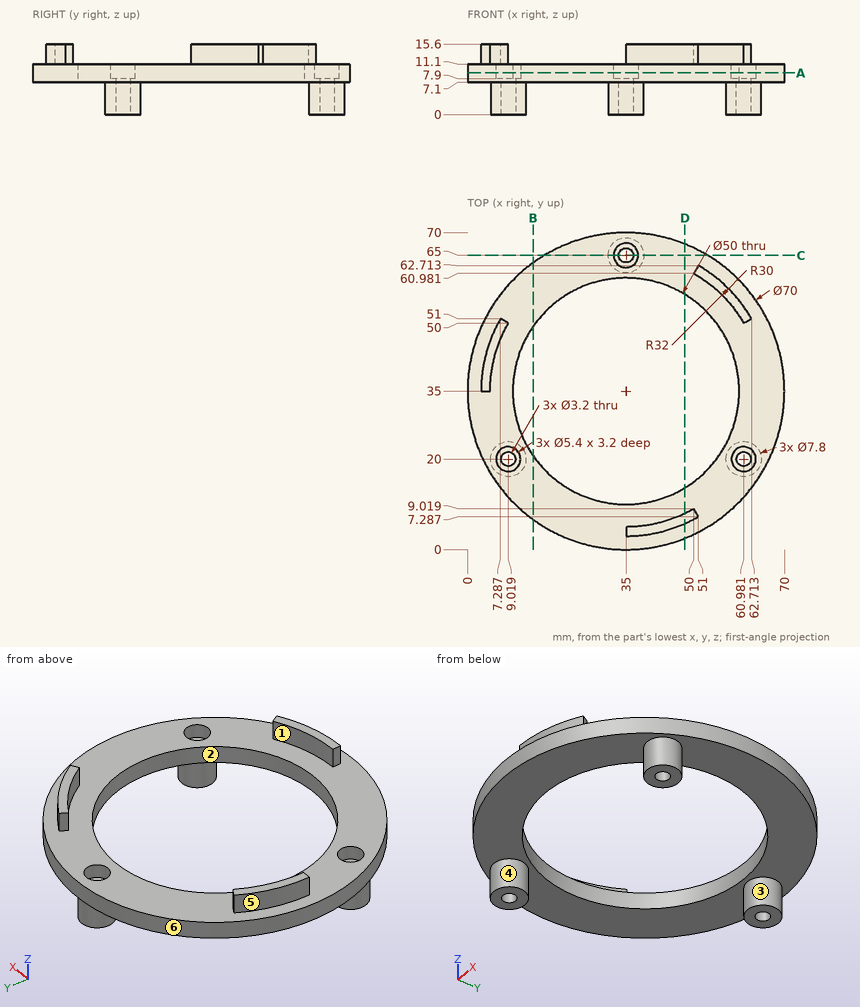
Drawing for the job (mm, zero at the part's lowest x, y, z). A direction names the side the tool comes from. Give positions to 0.01 mm unless a question says otherwise; leave off trailing zeros. Loops run counter-clockwise (first coordinate to the right, second up) from the corner with the lowest first, then second, coordinate; pieces in that order, holes last.
(1) Pin check, flat tips, straight feed: pin 1 (12 mm diameter, centred on x = 36.5, y = 12.5, fed in from +Z); pin 2 (8 mm diameter, centred on y = 45.5, z = 4, fed in from -X); pin 3 (1.6 mm diameter, centred on x = 8.5, y = 19, fed in from +Z). Stop position of each tip, or through.
Return value:
pin 1: stops at z = 11.1
pin 2: stops at x = 0.92
pin 3: stops at z = 7.9
(2) Drill centre lines: line 1 along Y through (x, z) = (35, 9.6); line 2 along Z through (x, y) = (62, 28.5); line 3 along Y through (x, z) = (35, 2.75). Where is each one in solid material? Low to high.
Return value:
line 1: y = 0 to 10, 60 to 62.3, 67.7 to 70
line 2: z = 7.1 to 11.1
line 3: y = 61.1 to 63.4, 66.6 to 68.9
(3) Band-saw the part on C-C (y = 65). Write the cut outline in (x, z).
Return value:
outline: (16.97, 7.1) - (31.1, 7.1) - (31.1, 0) - (33.4, 0) - (33.4, 7.9) - (32.3, 7.9) - (32.3, 11.1) - (16.97, 11.1) - close; (36.6, 0) - (38.9, 0) - (38.9, 7.1) - (53.03, 7.1) - (53.03, 11.1) - (37.7, 11.1) - (37.7, 7.9) - (36.6, 7.9) - close
(4) 3-axis set-ups, long thin cutter, end or side, ignore diameter. For the marked faces 4, 5 and 6: which of +Z, -Z, +X, -X, +Y, -Y reach the whole face in a straight line?
Return value:
face 4: -Z
face 5: +Z, -X, +Y
face 6: +Z, -Z
(5) Band-saw the part on B-B (x = 14.5). Write the cut outline in (y, z).
Return value:
outline: (6.63, 7.1) - (20.69, 7.1) - (20.69, 11.1) - (6.63, 11.1) - close; (49.31, 7.1) - (63.37, 7.1) - (63.37, 11.1) - (49.31, 11.1) - close
(6) Pull direction X, two halves, no side cores. Call the marked faces 1, 2 and 3: pulls with the +X half, pulls with the -X half, needs draft (parallel to the pull), parting line crosses it, or undercut.
Return value:
face 1: pulls with the -X half
face 2: undercut
face 3: parting line crosses it
(7) Band-saw the part on D-D (x = 48). Write the cut outline in (y, z).
Return value:
outline: (2.5, 7.1) - (13.65, 7.1) - (13.65, 11.1) - (7.96, 11.1) - (7.96, 15.6) - (5.76, 15.6) - (5.76, 11.1) - (2.5, 11.1) - close; (56.35, 7.1) - (67.5, 7.1) - (67.5, 11.1) - (56.35, 11.1) - close
(8) Band-saw the part on A-A (z = 9.25). Write the cut outline in (x, y), and give its area (3 significant figures).
Return value:
outline: circle Ø70 at (35, 35); hole circle Ø5.4 at (9.02, 20); hole circle Ø50 at (35, 35); hole circle Ø5.4 at (35, 65); hole circle Ø5.4 at (60.98, 20)
area: 1,820 mm2
